The figure shows three views and two pictorial views of one solid part (mm, origin at its lowest corner). Answer the questions. A direction names the side the tool comes from. Coordinates: 2 decimals unless noted, no trailing zeros. Loops run counter-clockwise (first coordinate to the right, second up) from the corner with the lowest first, then second, coordinate; pieces in that order, holes last.
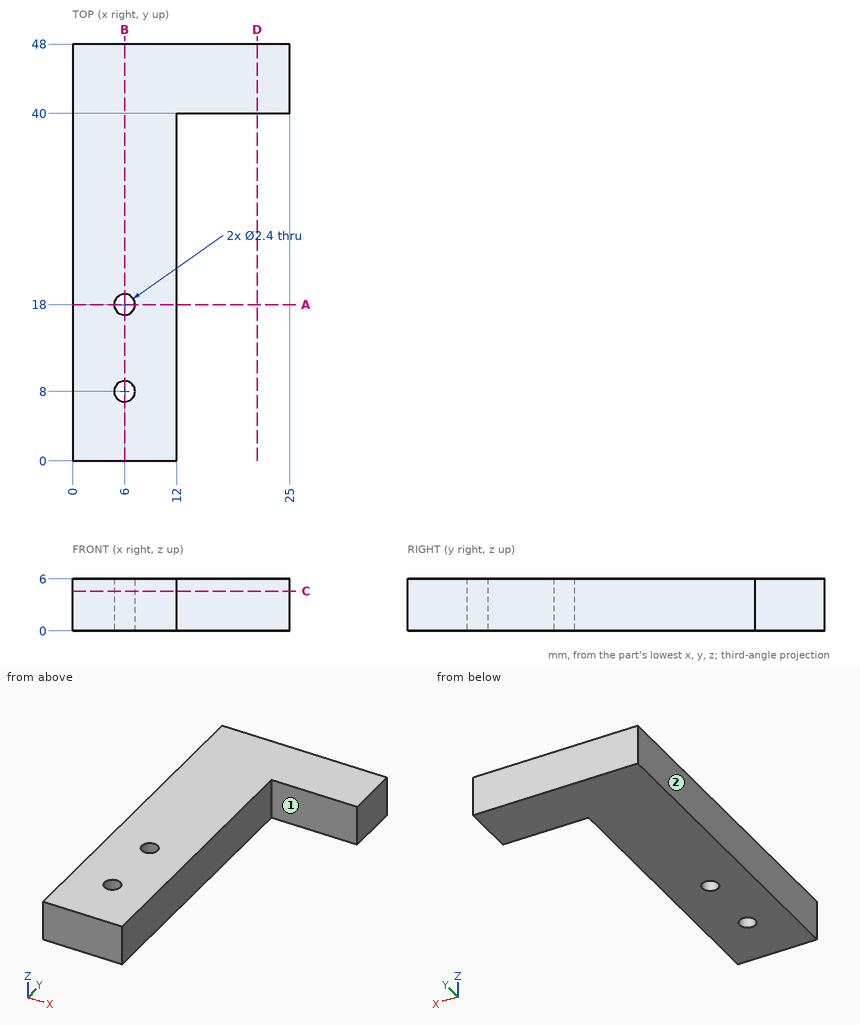
Q1. Which of the six approach directions +Z, -Z, +X, -X, +Y, -Y give full straight-line access (tool end or side, diameter ignored) to the marked faces 1 and 2?
Findings below:
face 1: +Z, -Z, +X, -Y
face 2: +Z, -Z, -X, +Y, -Y
Q2. Straight lines are drawn through the part: probe 1 along Y at (x, z) = (6, 2.3); probe 2 along X at (y, z) = (28, 3.1); probe 3 along Y at (x, z) = (22.75, 2.6). For each, find the intervals that lie inside material, in ascending order.
Findings below:
probe 1: y = 0 to 6.8, 9.2 to 16.8, 19.2 to 48
probe 2: x = 0 to 12
probe 3: y = 40 to 48
Q3. A cutting plane is placed at B-B (x = 6). Give the vertices of the cut face in (y, z), then the cut area to 3 significant figures.
Findings below:
outline: (0, 0) - (6.8, 0) - (6.8, 6) - (0, 6) - close; (9.2, 0) - (16.8, 0) - (16.8, 6) - (9.2, 6) - close; (19.2, 0) - (48, 0) - (48, 6) - (19.2, 6) - close
area: 259 mm2
Q4. Flat-ended cylindrical pins translate along their axes: pin 1 Ø3 at (x, z) = (16, 4) entering from -Y; pin 2 Ø3 at (y, z) = (13.5, 4) entering from +X; pin 3 Ø1.9 at (x, y) = (6, 8) entering from +Z. Find the tip coordinate at first contact, or state that the pin passes through.
Findings below:
pin 1: stops at y = 40
pin 2: stops at x = 12
pin 3: passes through
Q5. A cutting plane is placed at A-A (y = 18). Give the vertices of the cut face in (x, z).
Findings below:
outline: (0, 0) - (4.8, 0) - (4.8, 6) - (0, 6) - close; (7.2, 0) - (12, 0) - (12, 6) - (7.2, 6) - close
Q6. A cutting plane is placed at C-C (z = 4.6). Give the vertices of the cut face in (x, y), then the cut area to 3 significant figures.
Findings below:
outline: (0, 0) - (12, 0) - (12, 40) - (25, 40) - (25, 48) - (0, 48) - close; hole circle Ø2.4 at (6, 8); hole circle Ø2.4 at (6, 18)
area: 671 mm2
Q7. A cutting plane is placed at D-D (x = 21.25). Give the vertices of the cut face in (y, z).
Findings below:
outline: (40, 0) - (48, 0) - (48, 6) - (40, 6) - close
